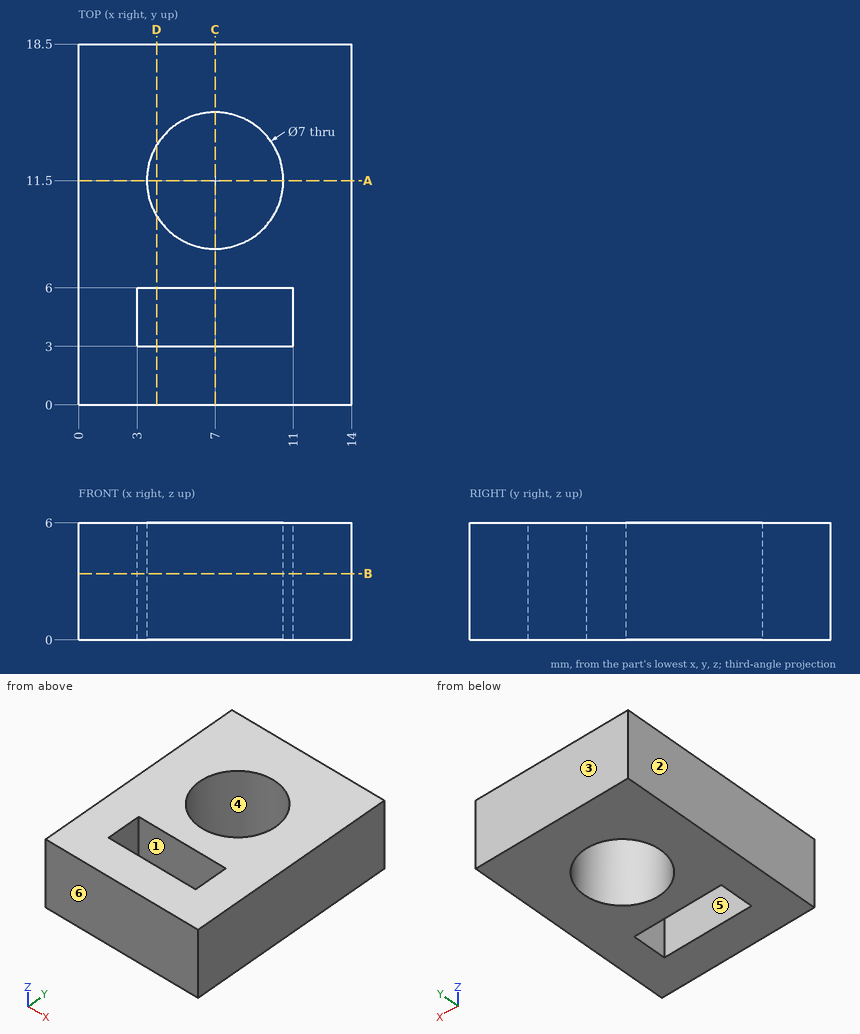
Answer from the drawing. Dimensions are ordinates in mm from the lowest x, y and z of the part. A direction names the side the tool comes from. Give positions to 0.01 mm unless a question says otherwise; leave off trailing zeros. Write each loop counter-clockwise with the first axis right and the second up, starting at its lowest first coordinate (ties: lowest second). Pieces come first, ordered by that corner, then holes. Notation, with made-up numbers: (63.5, -0.5) -> (79.5, -0.5) arc R7 cw to (79.5, 9.5) -> close; hole circle Ø4 at (-33.5, 71.25). An arc over 180 degrees is marked (long way). Use a Markdown table: item, result.
(1) Determine the mould class of the marked faces 1, 2, 3 and 4 for opening direction Y: released by +Y, released by -Y, zero draft, split by the parting line, or undercut.
Return value:
| item | result |
|---|---|
| face 1 | undercut |
| face 2 | zero draft |
| face 3 | released by +Y |
| face 4 | undercut |
(2) For the marked faces 5 and 6, determine the directions among +Z, -Z, +X, -X, +Y, -Y from which every point of the face is accessible in a straight line to the end or side of a thin tool.
Return value:
| item | result |
|---|---|
| face 5 | +Z, -Z |
| face 6 | +Z, -Z, +X, -X, -Y |
(3) Section C-C, the plane x = 7 is taken. Determine the outline of the cut face in (y, z), then the cut area to 3 significant figures.
Return value:
| item | result |
|---|---|
| outline | (0, 0) -> (3, 0) -> (3, 6) -> (0, 6) -> close; (6, 0) -> (8, 0) -> (8, 6) -> (6, 6) -> close; (15, 0) -> (18.5, 0) -> (18.5, 6) -> (15, 6) -> close |
| area | 51.0 mm2 |
(4) Section D-D, the plane x = 4 is taken. Determine the outline of the cut face in (y, z).
Return value:
| item | result |
|---|---|
| outline | (0, 0) -> (3, 0) -> (3, 6) -> (0, 6) -> close; (6, 0) -> (9.7, 0) -> (9.7, 6) -> (6, 6) -> close; (13.3, 0) -> (18.5, 0) -> (18.5, 6) -> (13.3, 6) -> close |
(5) Find the intervals of material crossed by probe 1 along Y at (x, z) = (7, 4.15); probe 2 along Y at (x, z) = (10, 5.65); probe 3 along X at (y, z) = (4, 4.35), in increasing order. Write a range as from..to.
Return value:
| item | result |
|---|---|
| probe 1 | 0..3, 6..8, 15..18.5 |
| probe 2 | 0..3, 6..9.7, 13.3..18.5 |
| probe 3 | 0..3, 11..14 |
(6) Section A-A, the plane y = 11.5 is taken. Determine the outline of the cut face in (x, z), then the cut area to 3 significant figures.
Return value:
| item | result |
|---|---|
| outline | (0, 0) -> (3.5, 0) -> (3.5, 6) -> (0, 6) -> close; (10.5, 0) -> (14, 0) -> (14, 6) -> (10.5, 6) -> close |
| area | 42.0 mm2 |
(7) Section B-B, the plane z = 3.4 is taken. Determine the outline of the cut face in (x, y).
Return value:
| item | result |
|---|---|
| outline | (0, 0) -> (14, 0) -> (14, 18.5) -> (0, 18.5) -> close; hole (3, 3) -> (11, 3) -> (11, 6) -> (3, 6) -> close; hole circle Ø7 at (7, 11.5) |
